Source: CAD feature listing. Evaluate the final solid. Frame: model axes, mm. Face numbers are marked on the shaded views. A direction names the side the tool comes from. Give positions to 0.01 mm unless a question says otherwise; leave off trailing zeros. Loops run counter-clockwise (first coordinate to the right, second up) from the corner with the lowest first, then second, coordinate; pieces in that order, holes last.
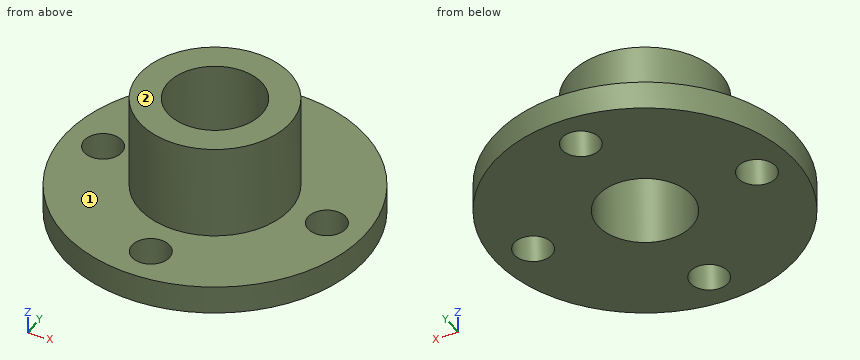
```python
from build123d import *

# Parameters (mm, degrees)
SKETCH_1_R          = 16
EXTRUDE_1_DEPTH     = 3
SKETCH_2_R          = 8
EXTRUDE_2_DEPTH     = 10
CUT_EXTRUDE_1_REACH = 28.096
SKETCH_3_R          = 5
SKETCH_3_R_2        = 2


with BuildPart() as part:
    # 草图1 → 凸台-拉伸1 (new body)
    with BuildSketch(Plane.XY):
        Circle(SKETCH_1_R)
    extrude(amount=EXTRUDE_1_DEPTH)

    # 草图2 → 凸台-拉伸2 (add)
    with BuildSketch(Plane.XY.offset(3)):
        Circle(SKETCH_2_R)
    extrude(amount=EXTRUDE_2_DEPTH)

    # 草图3 → 切除-拉伸1 (cut, up to next)
    with BuildSketch(Plane.XY.offset(13), mode=Mode.PRIVATE) as cut_extrude_1_sk1:
        Circle(SKETCH_3_R)
    cut_extrude_1_tool1 = extrude(cut_extrude_1_sk1.sketch, amount=-CUT_EXTRUDE_1_REACH, mode=Mode.PRIVATE) & part.part
    # 草图3 → 切除-拉伸1 (cut, up to next)
    with BuildSketch(Plane.XY.offset(13), mode=Mode.PRIVATE) as cut_extrude_1_sk2:
        with Locations((0, 12)):
            Circle(SKETCH_3_R_2)
    cut_extrude_1_tool2 = extrude(cut_extrude_1_sk2.sketch, amount=-CUT_EXTRUDE_1_REACH, mode=Mode.PRIVATE) & part.part
    # 草图3 → 切除-拉伸1 (cut, up to next)
    with BuildSketch(Plane.XY.offset(13), mode=Mode.PRIVATE) as cut_extrude_1_sk3:
        with Locations((12, 0)):
            Circle(SKETCH_3_R_2)
    cut_extrude_1_tool3 = extrude(cut_extrude_1_sk3.sketch, amount=-CUT_EXTRUDE_1_REACH, mode=Mode.PRIVATE) & part.part
    # 草图3 → 切除-拉伸1 (cut, up to next)
    with BuildSketch(Plane.XY.offset(13), mode=Mode.PRIVATE) as cut_extrude_1_sk4:
        with Locations((0, -12)):
            Circle(SKETCH_3_R_2)
    cut_extrude_1_tool4 = extrude(cut_extrude_1_sk4.sketch, amount=-CUT_EXTRUDE_1_REACH, mode=Mode.PRIVATE) & part.part
    # 草图3 → 切除-拉伸1 (cut, up to next)
    with BuildSketch(Plane.XY.offset(13), mode=Mode.PRIVATE) as cut_extrude_1_sk5:
        with Locations((-12, 0)):
            Circle(SKETCH_3_R_2)
    cut_extrude_1_tool5 = extrude(cut_extrude_1_sk5.sketch, amount=-CUT_EXTRUDE_1_REACH, mode=Mode.PRIVATE) & part.part
    add(cut_extrude_1_tool1.solids().sort_by_distance((0, 0, 13))[0], mode=Mode.SUBTRACT)
    add(cut_extrude_1_tool2.solids().sort_by_distance((0, 12, 13))[0], mode=Mode.SUBTRACT)
    add(cut_extrude_1_tool3.solids().sort_by_distance((12, 0, 13))[0], mode=Mode.SUBTRACT)
    add(cut_extrude_1_tool4.solids().sort_by_distance((0, -12, 13))[0], mode=Mode.SUBTRACT)
    add(cut_extrude_1_tool5.solids().sort_by_distance((-12, 0, 13))[0], mode=Mode.SUBTRACT)


solid = part.part
```
(1) Section C-C, the plane y = 11. Return the cut outline in (x, z).
A:
outline: (-11.62, 0) - (-1.73, 0) - (-1.73, 3) - (-11.62, 3) - close; (1.73, 0) - (11.62, 0) - (11.62, 3) - (1.73, 3) - close
(2) Section A-A, the plane y = 0. Return the cut outline in (x, z).
A:
outline: (-16, 0) - (-14, 0) - (-14, 3) - (-16, 3) - close; (-10, 0) - (-5, 0) - (-5, 13) - (-8, 13) - (-8, 3) - (-10, 3) - close; (5, 0) - (10, 0) - (10, 3) - (8, 3) - (8, 13) - (5, 13) - close; (14, 0) - (16, 0) - (16, 3) - (14, 3) - close
(3) Section D-D, the plane x = 12. Return the cut outline in (y, z).
A:
outline: (-10.58, 0) - (-2, 0) - (-2, 3) - (-10.58, 3) - close; (2, 0) - (10.58, 0) - (10.58, 3) - (2, 3) - close
(4) Reachability of the marked faces 1 and 2 from +Z, -Z, +X, -X, +Y, -Y: full face, straight path, thin tool, end or side. Return the list, or none.
A:
face 1: +Z
face 2: +Z, +X, -X, +Y, -Y
(5) First-contact query: pin 1 (6 mm diameter, centred on y = -12.5, z = 7, fed in from +X); pin 2 (5 mm diameter, centred on y = 6, z = 9.5, fed in from -X); pin 3 (8 mm diameter, centred on x = 13, y = 11.5, fed in from +Z). Flat tips, straight axial feed; report the tip coordinate or a pass-through.
A:
pin 1: passes through
pin 2: stops at x = -7.19
pin 3: stops at z = 3
(6) Ray query, line 1 along Y through (x, z) = (0, 3.75); line 2 along Z through (x, y) = (-10.5, -7); line 3 along Y through (x, z) = (1.5, 1.5). Return the intervals inside material, ascending.
A:
line 1: y = -8 to -5, 5 to 8
line 2: z = 0 to 3
line 3: y = -15.93 to -13.32, -10.68 to -4.77, 4.77 to 10.68, 13.32 to 15.93
